```python
from build123d import *

# Parameters (mm, degrees)
CORTE_EXTRUS_O1_REACH      = 110.839
CORTE_EXTRUS_O1_END_RADIUS = 21.5
PADR_OCIRCULAR1_COUNT      = 3


with BuildPart() as part:
    # Esboço1 → Revolução1 (revolve)
    with BuildSketch(Plane(origin=(0, 0, 0), x_dir=(0, 0, -1), z_dir=(1, 0, 0)), mode=Mode.PRIVATE) as revolu_o1_sk:
        with BuildLine():
            Line((-13.977542355, 71), (-10.977542355, 71))
            ThreePointArc((-10.977542355, 71), (-10.368780926, 70.79335334), (-10.011616529, 70.258819045))
            Line((-10.011616529, 70.258819045), (-0.102222521, 33.276457135))
            ThreePointArc((-0.102222521, 33.276457135), (-0.025665416, 32.891578577), (0, 32.5))
            Line((0, 32.5), (0, 26.5))
            ThreePointArc((0, 26.5), (0.146446609, 26.146446609), (0.5, 26))
            ThreePointArc((0.5, 26), (3.681980515, 24.681980515), (5, 21.5))
            Line((5, 21.5), (5, 20.5))
            Line((5, 20.5), (0.5, 20.5))
            Line((0.5, 20.5), (0.5, 18.5))
            Line((0.5, 18.5), (-37.5, 18.5))
            Line((-37.5, 18.5), (-37.5, 20.5))
            Line((-37.5, 20.5), (-42, 20.5))
            Line((-42, 20.5), (-42, 21.5))
            Line((-42, 21.5), (-2, 21.5))
            Line((-2, 21.5), (-2, 26.5))
            Line((-2, 26.5), (-2, 32.5))
            ThreePointArc((-2, 32.5), (-2.008555139, 32.630526192), (-2.034074174, 32.758819045))
            Line((-2.034074174, 32.758819045), (-11.744869343, 69))
            Line((-11.744869343, 69), (-13.977542355, 69))
            Line((-13.977542355, 69), (-13.977542355, 71))
        make_face()
    revolve(revolu_o1_sk.sketch.rotate(Axis((0, 0, 0), (0, 0, -1)), 90), axis=Axis((0, 0, 0), (0, 0, -1)))

    # Corte-extrusão1: up to this cylinder (the profile starts inside it)
    corte_extrus_o1_end = Plane(origin=(0, 0, 21.326762), z_dir=(0, 0, 1)) * Cylinder(CORTE_EXTRUS_O1_END_RADIUS, 265.678, mode=Mode.PRIVATE)
    # Esboço2 → Corte-extrusão1 (cut, up to the surface)
    with BuildSketch(Plane(origin=(0, 0, 0), x_dir=(0, 0, -1), z_dir=(1, 0, 0)), mode=Mode.PRIVATE) as corte_extrus_o1_sk1:
        with BuildLine():
            Line((-14.579629472, -7.776644394), (-31.494096646, -1.620281814))
            ThreePointArc((-31.494096646, -1.620281814), (-34.482459034, 4.788282007), (-28.073895213, 7.776644394))
            Line((-28.073895213, 7.776644394), (-11.159428039, 1.620281814))
            ThreePointArc((-11.159428039, 1.620281814), (-8.171065652, -4.788282007), (-14.579629472, -7.776644394))
        make_face()
    corte_extrus_o1_tool1 = extrude(corte_extrus_o1_sk1.sketch, amount=-CORTE_EXTRUS_O1_REACH, mode=Mode.PRIVATE) & corte_extrus_o1_end
    corte_extrus_o1 = corte_extrus_o1_tool1.solids().sort_by_distance((0, 0, 21.326762))[0]
    add(corte_extrus_o1, mode=Mode.SUBTRACT)

    # PadrãoCircular1: Corte-extrusão1 ×3 about axis
    padr_ocircular1_axis = Axis((0, 0, 0), (0, 0, 1))
    for i in range(1, PADR_OCIRCULAR1_COUNT):
        add(corte_extrus_o1.rotate(padr_ocircular1_axis, i * 360 / PADR_OCIRCULAR1_COUNT), mode=Mode.SUBTRACT)


solid = part.part
```
The listing builds one solid part. Answer for the finished solid, in the listing's coordinates (mm). A direction names the side the tool comes from. Give positions to 0.01 mm unless a question says otherwise; leave off trailing zeros. Order: outer loops, then holes, each group sorted by start corner. A loop starts at its lowest first (then second) coordinate and runs counter-clockwise, first axis right, second up. Notation, with made-up numbers: (45, 38.25) -> (87, 38.25) arc R29 cw to (87, 61.25) -> close; hole circle Ø6 at (-12, -36). An arc over 180 degrees is marked (long way). Write each question's results on one line, items separated by ' | '.
Q1. The part is cut by section A-A, the plane z = 19. Give the vertices of the cut face in (x, y).
Checked values:
outline: (-21.03, 4.47) -> (-17.95, 4.47) arc R18.5 cw to (3.38, 18.19) -> (4.96, 20.92) arc R21.5 ccw to start; (-20.6, -6.17) arc R21.5 ccw to (6.64, -20.45) -> (5.1, -17.78) arc R18.5 cw to (-17.44, -6.17) -> close; (12.85, 13.31) arc R18.5 cw to (14.06, -12.02) -> (15.64, -14.75) arc R21.5 ccw to (14.39, 15.97) -> close
Q2. Which of the six approach directions +Z, -Z, +X, -X, +Y, -Y give full straight-line access (tool end or side, diameter ignored) to faces 4 (the face through (-10.7, -15.3, -0.5)), 5 (the face through (13.646, -14.153, 22.918)), 6 (the face through (-21, 7, 2)), 7 (the face through (-19.08, -4.74, 22.92))?
Checked values:
face 4: -Z | face 5: -Y | face 6: +Z | face 7: -X
Q3. Determine the mould class of faces 1 (the face through (18.937, 7.852, 39.782)), 2 (the face through (0, 21, -5)), 3 (the face through (5.43, 18.89, 22.92)) for opening direction X: pulls with the +X half, pulls with the -X half, needs draft (parallel to the pull), parting line crosses it, or undercut.
Checked values:
face 1: undercut | face 2: needs draft | face 3: pulls with the +X half
Q4. Straight lines are drawn through the part: probe 1 along Y at (x, z) = (0, 12.75); probe 2 along Y at (x, z) = (0, 39.9); probe 3 along Z at (x, y) = (5.5, 21). For each, find the intervals that lie inside material, in ascending order. Write a range as from..to.
Checked values:
probe 1: y = -71..-69, -21.5..-18.5, 18.5..21.5, 69..71 | probe 2: y = -21.5..-20.5, 20.5..21.5 | probe 3: z = -5..2
Q5. Each of these flat-tipped pins is pushed along its axis until it touches: P1, Ø1, axis at x = 13.5, y = -54.5, coming from the +Z side; P2, Ø8, axis at y = 19, z = 15.5, coming from the +X side; P3, Ø12, axis at x = 42, z = 10, coming from the -Y side. Where does it stop, or does it pass through?
Checked values:
P1: stops at z = 8.43 | P2: stops at x = 69.33 | P3: stops at y = -61.15
